CAD build for the part. Positions are in the model's coordinates, mm. Face numbers are marked on the shaded views. A direction names the side the tool comes from. Coordinates: 2 decimals unless noted, no trailing zeros. Order: outer loops, then holes, each group sorted by start corner. A loop starts at its lowest first (then second) coordinate and runs counter-clockwise, first axis right, second up. Notation, with made-up numbers: M -16.75,30 L 6.25,30 A32 ccw 6.25,60 Z; hole C 59.5,50 d4. An arc over 180 degrees is marked long. Write item = value, one per line.
from build123d import *

# Parameters (mm, degrees)
F0_R     = 7.5
F1_DEPTH = 4
F2_R     = 5
F3_DEPTH = 100
F4_W     = 4
F4_H     = 4
F5_DEPTH = 20
F6_W     = 2.261252
F6_H     = 1
F7_DEPTH = 3


with BuildPart() as f1:
    # F0 (on Top) → F1 (new body)
    with BuildSketch(Plane.XY):
        Circle(F0_R)
    extrude(amount=F1_DEPTH)

    # F2 (on Top) → F3 (join)
    with BuildSketch(Plane.XY):
        Circle(F2_R)
    extrude(amount=F3_DEPTH)

    # F4 (on face) → F5 (join)
    with BuildSketch(Plane.XY.offset(100)):
        Rectangle(F4_W, F4_H)
    extrude(amount=F5_DEPTH)

    # F6 (on face) → F7 (cut)
    with BuildSketch(Plane.XY.offset(120)):
        with Locations((1.630626, 0)):
            Rectangle(F6_W, F6_H)
    extrude(amount=-F7_DEPTH, mode=Mode.SUBTRACT)


solid = f1.part
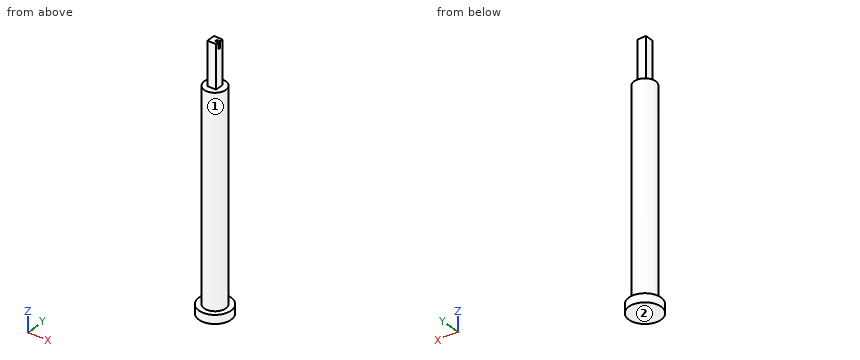
(1) Pin check, flat tips, straight feed: pin 1 Ø2 at (x, z) = (0.5, 105.5) entering from +Y; pin 2 Ø3 at (x, z) = (-1.5, 37.5) entering from +Y; pin 3 Ø1 at (y, z) = (3.5, 49.5) entering from +X. Stop position of each tip, or through.
Evaluation:
pin_1 = 2
pin_2 = 5
pin_3 = 4
(2) Wall check: line 1 (Z direction, x = -5, y = -1.75); line 2 (Z direction, x = -3, y = 3.5); line 3 (Y direction, x = -0.5, z = 23). Give the ranges that are in metal, low to high. Write a range as from..to.
Evaluation:
line_1 = 0..4
line_2 = 0..100
line_3 = -4.97..4.97
(3) Slice it at C-C, the plane z = 36. Write the cut outline in (x, y), then the cut area to 3 significant figures.
Evaluation:
outline = C 0,0 d10
area = 78.5 mm²
(4) Slice it at A-A, the plane y = 3.75. Write the cut outline in (x, z), then the cut area to 3 significant figures.
Evaluation:
outline = M -6.5,0 L 6.5,0 L 6.5,4 L 3.31,4 L 3.31,100 L -3.31,100 L -3.31,4 L -6.5,4 Z
area = 687 mm²
(5) Tool access for the marked faces 1 and 2: list every direction of +Z, -Z, +X, -X, +Y, -Y with a clear straight run to the whole face (end or side of a thin tool).
Evaluation:
face_1 = +Z
face_2 = -Z, +X, -X, +Y, -Y
